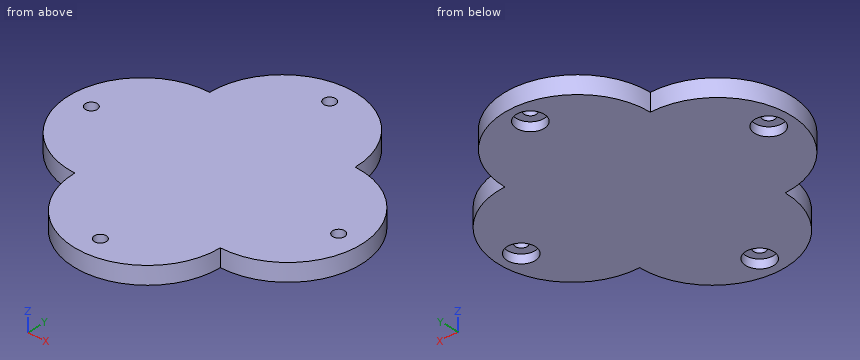
from build123d import *

# Parameters (mm, degrees)
IZIM1_R                     = 9.5
Y_KSEKLIK_EKSTR_ZYON1_DEPTH = 12
Y_KSEKLIK_EKSTR_ZYON2_START = -6
IZIM2_R                     = 9.5
IZIM2_R_2                   = 4.05
Y_KSEKLIK_EKSTR_ZYON2_DEPTH = 6


with BuildPart() as part:
    # Çizim1 → Yükseklik-Ekstrüzyon1 (new body)
    with BuildSketch(Plane.XY):
        with BuildLine():
            ThreePointArc((55.555555556, 45.593869732), (5.555555556, 95.593869732), (-44.444444444, 45.593869732))
            ThreePointArc((-44.444444444, 45.593869732), (-94.444444444, -4.406130268), (-44.444444444, -54.406130268))
            ThreePointArc((-44.444444444, -54.406130268), (5.555555556, -104.406130268), (55.555555556, -54.406130268))
            ThreePointArc((55.555555556, -54.406130268), (105.555555556, -4.406130268), (55.555555556, 45.593869732))
        make_face()
        with Locations((-79.444444444, -4.406130268)):
            Circle(IZIM1_R, mode=Mode.SUBTRACT)
        with Locations((5.555555556, 80.593869732)):
            Circle(IZIM1_R, mode=Mode.SUBTRACT)
        with Locations((90.555555556, -4.406130268)):
            Circle(IZIM1_R, mode=Mode.SUBTRACT)
        with Locations((5.555555556, -89.406130268)):
            Circle(IZIM1_R, mode=Mode.SUBTRACT)
    extrude(amount=Y_KSEKLIK_EKSTR_ZYON1_DEPTH)

    # Çizim2 → Yükseklik-Ekstrüzyon2 (add)
    # profile 1 of 4: a face of its own
    with BuildSketch(Plane.XY.offset(12).offset(Y_KSEKLIK_EKSTR_ZYON2_START)):
        with Locations((5.555555556, 80.593869732)):
            Circle(IZIM2_R)
        with Locations((5.555555556, 80.593869732)):
            Circle(IZIM2_R_2, mode=Mode.SUBTRACT)
    # profile 2 of 4: a face of its own
    with BuildSketch(Plane.XY.offset(12).offset(Y_KSEKLIK_EKSTR_ZYON2_START)):
        with Locations((90.555555556, -4.406130268)):
            Circle(IZIM2_R)
        with Locations((90.555555556, -4.406130268)):
            Circle(IZIM2_R_2, mode=Mode.SUBTRACT)
    # profile 3 of 4: a face of its own
    with BuildSketch(Plane.XY.offset(12).offset(Y_KSEKLIK_EKSTR_ZYON2_START)):
        with Locations((5.555555556, -89.406130268)):
            Circle(IZIM2_R)
        with Locations((5.555555556, -89.406130268)):
            Circle(IZIM2_R_2, mode=Mode.SUBTRACT)
    # profile 4 of 4: a face of its own
    with BuildSketch(Plane.XY.offset(12).offset(Y_KSEKLIK_EKSTR_ZYON2_START)):
        with Locations((-79.444444444, -4.406130268)):
            Circle(IZIM2_R)
        with Locations((-79.444444444, -4.406130268)):
            Circle(IZIM2_R_2, mode=Mode.SUBTRACT)
    extrude(amount=Y_KSEKLIK_EKSTR_ZYON2_DEPTH)


solid = part.part
Read the model definition and answer for the solid it produces. Units are mm, in the model's axes. Give positions to 0.01 mm unless a question says otherwise; leave off trailing zeros. Write each loop counter-clockwise with the first axis right and the second up, starting at its lowest first coordinate (ties: lowest second). Pieces come first, ordered by that corner, then holes. Notation, with made-up numbers: (-19, 48.25) - (12, 48.25) arc R11 cw to (12, 52.25) - close; hole circle Ø4 at (44, 55.5). An arc over 180 degrees is marked (long way). Answer in a Markdown table with one row per item. Add a question column.
Item 1: Find the intervals of material crossed by L1, parallel to Y at x = 9, z = 1; L2, parallel to Y at x = -75.5, z = 2; L3, parallel to Y at x = 92.5, z = 9, in increasing order.
Item 2: Section C-C, the plane y = 33.5 is taken. Write down the section's boundary in (x, z), and give its area (3 significant figures).
Item 3: Section A-A, the plane z = 8.75 is taken. Write down the section's boundary in (x, y), and give its area (3 significant figures).
Item 4: Flat-ended cylindrical pins translate along their axes: P1, Ø17, axis at x = 5.56, y = -89.41, coming from the -Z side; P2, Ø4, axis at x = 65, y = 4.5, coming from the -Z side; P3, Ø2, axis at y = 53, z = 2.5, coming from the -X side; P4, Ø2, axis at x = -7, z = 9, coming from the -Y side. Find the tip coordinate at first contact, or state that the pin passes through.
Item 5: Section B-B, the plane x = 92 is taken. Write down the section's boundary in (y, z), and give its area (3 significant figures).
Item 6: Section D-D, the plane x = 48 is taken. Write down the section's boundary in (y, z), and give its area (3 significant figures).
Recorded:
| question | item | result |
|---|---|---|
| 1 | L1 | y = -104.29 to -98.26, -80.55 to 71.74, 89.45 to 95.48 |
| 1 | L2 | y = -43.59 to -13.05, 4.24 to 34.78 |
| 1 | L3 | y = -38.1 to -7.96, -0.85 to 29.29 |
| 2 | outline | (-77.05, 0) - (88.16, 0) - (88.16, 12) - (-77.05, 12) - close |
| 2 | area | 1,980 mm2 |
| 3 | outline | (-44.44, -54.41) arc R50 ccw to (55.56, -54.41) arc R50 ccw to (55.56, 45.59) arc R50 ccw to (-44.44, 45.59) arc R50 ccw to start; hole circle Ø8.1 at (-79.44, -4.41); hole circle Ø8.1 at (5.56, -89.41); hole circle Ø8.1 at (5.56, 80.59); hole circle Ø8.1 at (90.56, -4.41) |
| 3 | area | 25,500 mm2 |
| 4 | P1 | stops at z = 6 |
| 4 | P2 | stops at z = 0 |
| 4 | P3 | stops at x = -44.03 |
| 4 | P4 | stops at y = -103.05 |
| 5 | outline | (-38.64, 0) - (-13.8, 0) - (-13.8, 6) - (-8.19, 6) - (-8.19, 12) - (-38.64, 12) - close; (-0.62, 6) - (4.98, 6) - (4.98, 0) - (29.83, 0) - (29.83, 12) - (-0.62, 12) - close |
| 5 | area | 663 mm2 |
| 6 | outline | (-80.83, 0) - (72.02, 0) - (72.02, 12) - (-80.83, 12) - close |
| 6 | area | 1,830 mm2 |
